Part print with two shaded views. Sizes in mm from the minimum x, y, z corner. A direction names the side the tool comes from. Round coordinates to 2 decimals unless told otherwise and drop trailing zeros. Write each loop counter-clockwise with the first axis right and the second up, starting at its lowest first coordinate (ties: lowest second). Pieces come first, ordered by that corner, then holes. Notation, with made-up numbers: (4.5, 19) -> (47.5, 19) arc R31 ccw to (47.5, 45) -> close; hole circle Ø7 at (88.5, -22). An arc over 180 degrees is marked (long way). Answer in a Markdown table with one row per item.
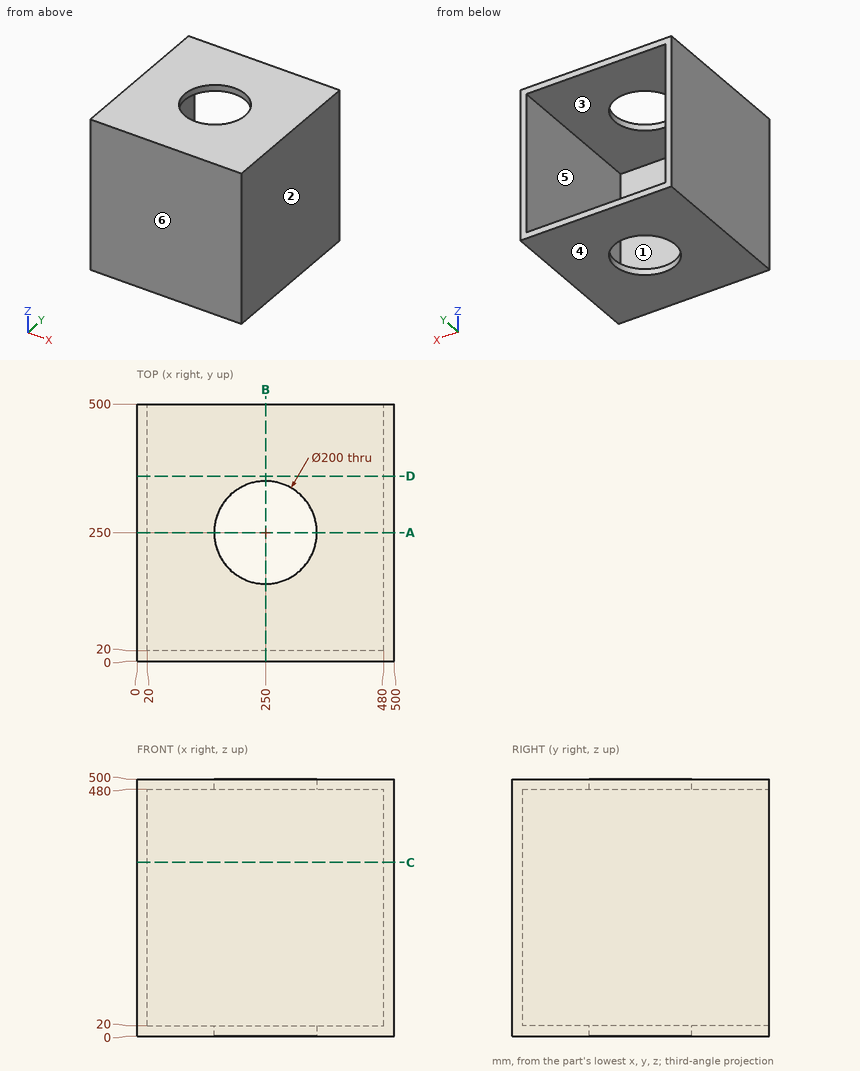
Q1. Saw through at B-B on x = 250. Write the cut outline in (y, z).
A:
| item | result |
|---|---|
| outline | (0, 0) -> (150, 0) -> (150, 20) -> (20, 20) -> (20, 480) -> (150, 480) -> (150, 500) -> (0, 500) -> close; (350, 0) -> (500, 0) -> (500, 20) -> (350, 20) -> close; (350, 480) -> (500, 480) -> (500, 500) -> (350, 500) -> close |
Q2. Saw through at D-D on y = 359.5. Write the cut outline in (x, z).
A:
| item | result |
|---|---|
| outline | (0, 0) -> (500, 0) -> (500, 500) -> (0, 500) -> close; hole (20, 20) -> (480, 20) -> (480, 480) -> (20, 480) -> close |
Q3. Wall check: line 1 (Y direction, x = 250, z = 485); line 2 (X direction, y = 192.5, z = 393.5). Give the ranges that are in metal, low to high. Write a range as [from, to].
A:
| item | result |
|---|---|
| line 1 | [0, 150], [350, 500] |
| line 2 | [0, 20], [480, 500] |
Q4. Which spindle directions (+Z, -Z, +X, -X, +Y, -Y) get a long thin tool onto all of the face, cutting with end or side? Do the marked faces 5 and 6. Say none if no direction does.
A:
| item | result |
|---|---|
| face 5 | +Y |
| face 6 | +Z, -Z, +X, -X, -Y |
Q5. Two-plate mould, pull along Z, no slides. Class the marked faces 1, 2, 3 and 4: released by +Z, released by -Z, zero draft, split by the parting line, or undercut.
A:
| item | result |
|---|---|
| face 1 | undercut |
| face 2 | zero draft |
| face 3 | undercut |
| face 4 | released by -Z |
Q6. Saw through at A-A on y = 250. Write the cut outline in (x, z), plus the area to 3 significant figures.
A:
| item | result |
|---|---|
| outline | (0, 0) -> (150, 0) -> (150, 20) -> (20, 20) -> (20, 480) -> (150, 480) -> (150, 500) -> (0, 500) -> close; (350, 0) -> (500, 0) -> (500, 500) -> (350, 500) -> (350, 480) -> (480, 480) -> (480, 20) -> (350, 20) -> close |
| area | 30,400 mm² |
Q7. Saw through at C-C on z = 338. Write the cut outline in (x, y).
A:
| item | result |
|---|---|
| outline | (0, 0) -> (500, 0) -> (500, 500) -> (480, 500) -> (480, 20) -> (20, 20) -> (20, 500) -> (0, 500) -> close |
